```python
from build123d import *

# Parameters (mm, degrees)
SKETCH1_R                = 7.5
SKETCH1_R_2              = 2.3241
BOSS_EXTRUDE1_DEPTH      = 2.794
SKETCH2_R                = 2.3241
BOSS_EXTRUDE2_DEPTH      = 0.254
BOSS_EXTRUDE3_DEPTH      = 1.651
BOSS_EXTRUDE4_START      = 2.286
SKETCH4_R                = 7.5
BOSS_EXTRUDE4_DEPTH      = 2.286
FILLET1_R                = 0.254
FILLET2_R                = 0.127
FILLET3_R                = 0.4
SKETCH6_W                = 4.02205745
SKETCH6_H                = 1.558094328
BOSS_EXTRUDE5_DEPTH      = 2.54
BOSS_EXTRUDE6_DEPTH      = 2.413
BOSS_EXTRUDE6_DEPTH_BACK = 2.413
CUT_EXTRUDE2_START       = -4
SKETCH5_R                = 6.3875
SKETCH5_R_2              = 2.3241
CUT_EXTRUDE2_DEPTH       = 4


with BuildPart() as part:
    # Sketch1 → Boss-Extrude1 (new body)
    with BuildSketch(Plane(origin=(0, 0, 0), x_dir=(1, 0, 0), z_dir=(0, 1, 0))):
        with Locations(Location((0, 0, 0), (0, 0, 270))):
            Circle(SKETCH1_R)
        with Locations(Location((0, 0, 0), (0, 0, 270))):
            Circle(SKETCH1_R_2, mode=Mode.SUBTRACT)
    extrude(amount=BOSS_EXTRUDE1_DEPTH)

    # Sketch2 → Boss-Extrude2 (add)
    with BuildSketch(Plane.XZ):
        with Locations(Location((0, 0, 0), (0, 0, 270))):
            Circle(SKETCH2_R)
    extrude(amount=-BOSS_EXTRUDE2_DEPTH)

    # Sketch3 → Boss-Extrude3 (add)
    with BuildSketch(Plane(origin=(0, 0.254, 0), x_dir=(1, 0, 0), z_dir=(0, 1, 0))):
        with BuildLine():
            Line((-0.495805164, 1.156686678), (0.614449488, 1.120298857))
            ThreePointArc((0.614449488, 1.120298857), (0.708812351, 1.091670316), (0.776218716, 1.01969584))
            Line((0.776218716, 1.01969584), (1.299833265, 0.039993196))
            ThreePointArc((1.299833265, 0.039993196), (1.322221652, -0.056041711), (1.293593111, -0.150404573))
            Line((1.293593111, -0.150404573), (0.706953007, -1.093719397))
            ThreePointArc((0.706953007, -1.093719397), (0.634978532, -1.161125762), (0.538943625, -1.183514149))
            Line((0.538943625, -1.183514149), (-0.571311028, -1.147126328))
            ThreePointArc((-0.571311028, -1.147126328), (-0.66567389, -1.118497787), (-0.733080255, -1.046523312))
            Line((-0.733080255, -1.046523312), (-1.256694804, -0.066820667))
            ThreePointArc((-1.256694804, -0.066820667), (-1.279083191, 0.02921424), (-1.25045465, 0.123577102))
            Line((-1.25045465, 0.123577102), (-0.663814546, 1.066891925))
            ThreePointArc((-0.663814546, 1.066891925), (-0.591840071, 1.134298291), (-0.495805164, 1.156686678))
        make_face()
    extrude(amount=BOSS_EXTRUDE3_DEPTH)

    # Sketch4 → Boss-Extrude4 (add)
    with BuildSketch(Plane.XZ.offset(BOSS_EXTRUDE4_START)):
        with Locations(Location((0, 0, 0), (0, 0, 270))):
            Circle(SKETCH4_R)
    extrude(amount=-BOSS_EXTRUDE4_DEPTH)

    # Fillet1
    fillet1_edges = [part.edges().sort_by_distance(p)[0] for p in [
        (0, 0.254, -2.3241),
        (0.708812351, 0.254, -1.091670316),
        (0.059322162, 0.254, -1.138492768),
        (-0.591840071, 0.254, -1.134298291),
        (-0.957134598, 0.254, -0.595234514),
        (-1.279083191, 0.254, -0.02921424),
        (-0.99488753, 0.254, 0.556671989),
        (-0.66567389, 0.254, 1.118497787),
        (-0.016183701, 0.254, 1.165320239),
        (0.634978532, 0.254, 1.161125762),
        (1.000273059, 0.254, 0.622061985),
        (1.322221652, 0.254, 0.056041711),
        (1.038025991, 0.254, -0.529844518),
    ]]
    fillet(fillet1_edges, radius=FILLET1_R)

    # Fillet2
    fillet2_edges = [part.edges().sort_by_distance(p)[0] for p in [
        (0.708812351, 1.905, -1.091670316),
        (0.059322162, 1.905, -1.138492768),
        (-0.591840071, 1.905, -1.134298291),
        (-0.957134598, 1.905, -0.595234514),
        (-1.279083191, 1.905, -0.02921424),
        (-0.99488753, 1.905, 0.556671989),
        (-0.66567389, 1.905, 1.118497787),
        (-0.016183701, 1.905, 1.165320239),
        (0.634978532, 1.905, 1.161125762),
        (1.000273059, 1.905, 0.622061985),
        (1.322221652, 1.905, 0.056041711),
        (1.038025991, 1.905, -0.529844518),
    ]]
    fillet(fillet2_edges, radius=FILLET2_R)

    # Fillet3
    fillet3_edges = [part.edges().sort_by_distance(p)[0] for p in [
        (0, 2.794, -7.5),
    ]]
    fillet(fillet3_edges, radius=FILLET3_R)

    # Sketch6 → Boss-Extrude5 (add)
    with BuildSketch(Plane.XZ.offset(2.286)):
        Rectangle(SKETCH6_W, SKETCH6_H)
    extrude(amount=BOSS_EXTRUDE5_DEPTH)

    # Sketch7 → Boss-Extrude6 (add, two sides: drawn at the far end of the back side and taken through both)
    with BuildSketch(Plane(origin=(0, 0, 0), x_dir=(-1, 0, 0), z_dir=(0, 0, -1)).offset(-BOSS_EXTRUDE6_DEPTH_BACK)):
        with BuildLine():
            Line((8.999999188, -2.286), (-8.999999188, -2.286))
            ThreePointArc((-8.999999188, -2.286), (-9.707105969, -2.578893219), (-9.999999188, -3.286))
            Line((-9.999999188, -3.286), (-9.999999188, -4.398115656))
            ThreePointArc((-9.999999188, -4.398115656), (-9.660822486, -5.148657173), (-8.873374049, -5.390066297))
            ThreePointArc((-8.873374049, -5.390066297), (0, -4.826), (8.873374049, -5.390066297))
            ThreePointArc((8.873374049, -5.390066297), (9.660822486, -5.148657173), (9.999999188, -4.398115656))
            Line((9.999999188, -4.398115656), (9.999999188, -3.286))
            ThreePointArc((9.999999188, -3.286), (9.707105969, -2.578893219), (8.999999188, -2.286))
        make_face()
    extrude(amount=BOSS_EXTRUDE6_DEPTH + BOSS_EXTRUDE6_DEPTH_BACK)

    # Sketch5 → Cut-Extrude2 (cut)
    # profile 1 of 2: a face of its own
    with BuildSketch(Plane(origin=(0, 2.794, 0), x_dir=(1, 0, 0), z_dir=(0, 1, 0)).offset(CUT_EXTRUDE2_START)):
        with Locations(Location((0, 0, 0), (0, 0, 270))):
            Circle(SKETCH5_R)
        Circle(SKETCH5_R_2, mode=Mode.SUBTRACT)
    # profile 2 of 2: a face of its own
    with BuildSketch(Plane(origin=(0, 2.794, 0), x_dir=(1, 0, 0), z_dir=(0, 1, 0)).offset(CUT_EXTRUDE2_START)):
        Circle(SKETCH5_R_2)
    extrude(amount=CUT_EXTRUDE2_DEPTH, mode=Mode.SUBTRACT)

    # Sketch11 → Revolve3 (revolve)
    with BuildSketch(Plane(origin=(0, 0, 0), x_dir=(-1, 0, 0), z_dir=(0, 0, -1)), mode=Mode.PRIVATE) as revolve3_sk:
        Polygon((-7.101227429, -2.286), (-7.5, -2.286), (0, -4.826), (0, -2.286), align=None)
    revolve(revolve3_sk.sketch.rotate(Axis((0, -1.206, 0), (0, 1, 0)), 18.767781972), axis=Axis((0, -1.206, 0), (0, 1, 0)))


solid = part.part
```
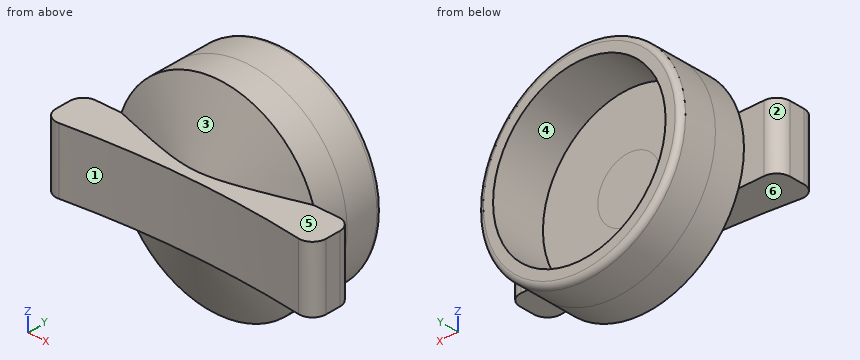
The model under review builds one solid part; all positions refer to its coordinate system, in mm. Face numbers are marked on the shaded views. A direction names the side the tool comes from. Give positions to 0.01 mm unless a question says otherwise; leave off trailing zeros. Write each loop counter-clockwise with the first axis right and the second up, starting at its lowest first coordinate (ties: lowest second). Pieces come first, ordered by that corner, then holes. Notation, with made-up numbers: (51, 11) -> (60, 11) arc R17 ccw to (60, 25) -> close; hole circle Ø8 at (69, -35.5). An arc over 180 degrees is marked (long way). Answer in a Markdown table with one row per item.
1) Clearance check with flat-ended pins moving along their axes: P1, Ø6, axis at x = 0.5, z = -1, coming from the +Y side; P2, Ø2, axis at y = 0.5, z = -6, coming from the -X side; P3, Ø2, axis at x = -7, y = -1, coming from the -Z side. State where each tip first meets the part, or that it passes through.
Worked answers:
| item | result |
|---|---|
| P1 | y = -1.21 |
| P2 | x = -5.59 |
| P3 | z = -4.5 |
2) Add section C-C on y = -2.5. State the section outline as (x, z) points.
Worked answers:
| item | result |
|---|---|
| outline | (-9.62, -2.41) -> (-6.43, -2.41) arc R6.87 ccw to (6.43, -2.41) -> (9.62, -2.41) -> (9.62, 2.41) -> (6.43, 2.41) arc R6.87 ccw to (-6.43, 2.41) -> (-9.62, 2.41) -> close |
3) For L1, parallel to X at y = 1.55, z = 0; L2, parallel to Z at x = 1.75, y = -4.5; L3, parallel to Z at x = 4, y = 0, list the stretches that pass through material, from the lowest coordinate up. Write a range as [from, to].
Worked answers:
| item | result |
|---|---|
| L1 | [-7.5, -6.39], [6.39, 7.5] |
| L2 | [-2.41, 2.41] |
| L3 | [-6.34, -4.98], [4.98, 6.34] |
4) Add section B-B on z = 0. State the section outline as (x, y) points, plus the area to 3 significant figures.
Worked answers:
| item | result |
|---|---|
| outline | (-10, -4.4) arc R1 ccw to (-8.87, -5.39) arc R70.08 cw to (8.87, -5.39) arc R1 ccw to (10, -4.4) -> (10, -3.29) arc R1 ccw to (9, -2.29) -> (7.5, -2.29) -> (7.5, 2.39) arc R0.4 ccw to (7.1, 2.79) -> (6.39, 2.79) -> (6.39, -1.21) -> (-6.39, -1.21) -> (-6.39, 2.79) -> (-7.1, 2.79) arc R0.4 ccw to (-7.5, 2.39) -> (-7.5, -2.29) -> (-9, -2.29) arc R1 ccw to (-10, -3.29) -> close |
| area | 79.6 mm² |
5) Add section A-A on x = 0. State the section outline as (y, z) points.
Worked answers:
| item | result |
|---|---|
| outline | (-4.83, -2.41) -> (-4.01, -2.41) -> (-2.29, -7.5) -> (2.39, -7.5) arc R0.4 ccw to (2.79, -7.1) -> (2.79, -6.39) -> (-1.21, -6.39) -> (-1.21, 6.39) -> (2.79, 6.39) -> (2.79, 7.1) arc R0.4 ccw to (2.39, 7.5) -> (-2.29, 7.5) -> (-4.01, 2.41) -> (-4.83, 2.41) -> close |
6) Add section D-D on y = -0.75. State the section outline as (x, z) points (1 decimal), plus the area to 3 significant figures.
Worked answers:
| item | result |
|---|---|
| outline | circle Ø15 at (0, 0); hole circle Ø12.8 at (0, 0) |
| area | 48.5 mm² |
7) Mouldability with a two-part tool opening along X and no side actions: class the marked faces 1, 2, 3 and 4 as +X half, -X half, draft (parallel to the pull), parting line (faces both ways), or undercut.
Worked answers:
| item | result |
|---|---|
| face 1 | undercut |
| face 2 | -X half |
| face 3 | parting line |
| face 4 | undercut |
8) Tool access review of the marked faces 5 and 6: name each direction out of +Z, -Z, +X, -X, +Y, -Y from which nothing blocks a thin tool from reaching the whole face with its end or side.
Worked answers:
| item | result |
|---|---|
| face 5 | +Z, -Y |
| face 6 | -Z, -Y |
